```python
from build123d import *

# Parameters (mm, degrees)
SKETCH1_R           = 3
BOSS_EXTRUDE1_DEPTH = 5
CHAMFER2_SIZE       = 0.2


with BuildPart() as part:
    # Sketch1 → Boss-Extrude1 (new body)
    with BuildSketch(Plane(origin=(0, 0, 0), x_dir=(1, 0, 0), z_dir=(0, 1, 0))):
        Polygon((-4.241992166, -4.202035335), (1.518073264, -5.774690646), (5.760065431, -1.572655311), (4.241992166, 4.202035335), (-1.518073264, 5.774690646), (-5.760065431, 1.572655311), align=None)
        with Locations(Location((0, 0, 0), (0, 0, 270))):
            Circle(SKETCH1_R, mode=Mode.SUBTRACT)
    extrude(amount=BOSS_EXTRUDE1_DEPTH)

    # Chamfer2
    chamfer2_edges = [part.edges().sort_by_distance(p)[0] for p in [
        (3.639069348, 5, 3.673672979),
        (5.001028798, 5, -1.314690012),
        (1.361959451, 5, -4.98836299),
        (-3.639069348, 5, -3.673672979),
        (-5.001028798, 5, 1.314690012),
        (-3.639069348, 0, -3.673672979),
        (1.361959451, 0, -4.98836299),
        (5.001028798, 0, -1.314690012),
        (-1.361959451, 5, 4.98836299),
        (3.639069348, 0, 3.673672979),
        (-1.361959451, 0, 4.98836299),
        (-5.001028798, 0, 1.314690012),
    ]]
    chamfer(chamfer2_edges, length=CHAMFER2_SIZE)


solid = part.part
```
The listing builds one solid part. Answer for the finished solid, in the listing's coordinates (mm). Give positions to 0.01 mm unless a question says otherwise; leave off trailing zeros. Order: outer loops, then holes, each group sorted by start corner. A loop starts at its lowest first (then second) coordinate and runs counter-clockwise, first axis right, second up. Notation, with made-up numbers: (52, 61.5) - (80, 61.5) arc R17 cw to (80, 94.5) - close; hole circle Ø5 at (74.5, 56.5). An arc over 180 degrees is marked (long way). Answer in a Markdown table with one row per item. Add a question column.
Q1. The part is cut by section A-A (x = 2.75). Determine the outline of the cut face in (y, z), then the cut area to 3 significant figures.
Q2. Find the intervals of material crossed by line 1 along Z through (x, y) = (2.25, 2.3); line 2 along Z through (x, y) = (-2.75, 2.3); line 3 along X through (y, z) = (3.6, 0), in increasing order. Write a range as [from, to].
Q3. For a pull along Z with two mould halves and no side action, classify faces 1 (the flat face through (3.61, 2.47, 3.7)), 2 (the cylindrical face through (0.9, 2.46, 2.86)), 3 (the flat face through (-3, 5, -3)), 4 (the flat face through (-3.61, 2.47, -3.7)) as released by +Z, released by -Z, zero draft, split by the parting line, or undercut.
Q4. The part is cut by section D-D (z = 4.5). Determine the outline of the cut face in (x, y).
Q5. The part is cut by section B-B (z = 0). Determine the outline of the cut face in (x, y), then the cut area to 3 significant figures.
Q6. The part is cut by section C-C (y = 4.35). Determine the outline of the cut face in (x, z), then the cut area to 3 significant figures.
Q7. Given P1, Ø1, axis at x = -2.5, z = -0.5, coming from the -Y side; P2, Ø1.5, axis at y = 2, z = -1.5, coming from the +X side; P3, Ø1.5, axis at y = 1, z = -4.5, coming from the -X side; P4, Ø2, axis at x = 4.5, y = 2.5, coming from the -Z side, each flat-ended and moving along its own axis, determine where each tip first touches the part or whether it passes through.
Determined:
| question | item | result |
|---|---|---|
| 1 | outline | (0, -4.4) - (0.2, -4.61) - (4.8, -4.61) - (5, -4.4) - (5, -1.2) - (0, -1.2) - close; (0, 1.2) - (5, 1.2) - (5, 4.27) - (4.8, 4.55) - (0.2, 4.55) - (0, 4.27) - close |
| 1 | area | 33.7 mm² |
| 2 | line 1 | z = [-4.75, -1.98], [1.98, 5.05] |
| 2 | line 2 | z = [-4.55, -1.2], [1.2, 4.61] |
| 2 | line 3 | x = [-5.35, -3], [3, 5.35] |
| 3 | face 1 | released by +Z |
| 3 | face 2 | undercut |
| 3 | face 3 | zero draft |
| 3 | face 4 | released by -Z |
| 4 | outline | (-3.15, 0.2) - (-2.39, 0) - (2.52, 0) - (2.8, 0.2) - (2.8, 4.8) - (2.52, 5) - (-2.39, 5) - (-3.15, 4.8) - close |
| 5 | outline | (-5.35, 0.2) - (-5.14, 0) - (-3, 0) - (-3, 5) - (-5.14, 5) - (-5.35, 4.8) - close; (3, 0) - (5.14, 0) - (5.35, 0.2) - (5.35, 4.8) - (5.14, 5) - (3, 5) - close |
| 5 | area | 23.4 mm² |
| 6 | outline | (-5.76, -1.57) - (-1.52, -5.77) - (4.24, -4.2) - (5.76, 1.57) - (1.52, 5.77) - (-4.24, 4.2) - close; hole circle Ø6 at (0, 0) |
| 6 | area | 64.4 mm² |
| 7 | P1 | stops at y = 0 |
| 7 | P2 | stops at x = 5.15 |
| 7 | P3 | stops at x = -3.56 |
| 7 | P4 | stops at z = -4.4 |
